Geometry: final body of the model. Coordinates: model frame, mm. A direction names the side the tool comes from. Give positions to 0.01 mm unless a question says otherwise; leave off trailing zeros. Order: outer loops, then holes, each group sorted by start corner. A loop starts at its lowest first (then second) coordinate and runs counter-clockwise, first axis right, second up. Notation, with made-up numbers: (-8, -5) -> (25, -5) arc R23 ccw to (25, 12) -> close; hole circle Ø4 at (48, -24). An arc over 180 degrees is marked (long way). Answer in a Markdown table with one row per item. Add a question column.
Q1. Cut plane C-C on z = 63. Return the cut outline in (x, y) (3 decimals), and give its area (3 significant figures).
Q2. Set-up query: faces 4 (the face through (25.4, 32, 6)), 5 (the face through (-12.827, 0, 63)), 6 (the face through (35, 25.4, 63)), 7 (the face through (-35, 25.4, 63)), 8 (the face through (38, 31, 118.745)). Return all of +Z, -Z, +X, -X, +Y, -Y with unobstructed straight access to the full face (end or side cutting, diameter ignored); none if empty.
Q3. Cut plane A-A on y = 2. Return the cut outline in (x, z).
Q4. Line query: line 1 along Z through (x, y) = (28.5, 60) (3 decimals); line 2 along X through (y, z) = (-3.5, 27); line 3 along X through (y, z) = (18, 77.5). Output: solid intervals per line, ascending. Write a range as from..to.
Q5. Pull-direction query (X, two-part tool) for faces 1 (the face through (0, 12.7, 63)), 2 (the face through (25.4, 32, 121)), 3 (the face through (-15, -12.7, 63)); classes: +X half, -X half, draft (parallel to the pull), parting line (faces both ways), or undercut.
Q6. Cut plane B-B on x = -38.5. Return the cut outline in (y, z) (3 decimals).
Q7. Contact query for flat-ended pins moving along their axis: P1, Ø1.5, axis at x = 40, z = 122.5, coming from the +Y side (3 decimals); P2, Ø5, axis at x = -31.5, z = 72, coming from the -Y side; P3, Ø7.5, axis at y = -1, z = 79, coming from the +X side. Output: stop coordinate, or through.
Q8. Cut plane D-D on x = 42. Return the cut outline in (y, z) (1 decimal), and give its area (3 significant figures).
from build123d import *

# Parameters (mm, degrees)
BOSS_EXTRUDE1_DEPTH = 127
SKETCH5_W           = 101.6
SKETCH5_H           = 127
BOSS_EXTRUDE3_DEPTH = 3.175
FILLET1_R           = 2.54
SKETCH6_W           = 101.6
SKETCH6_H           = 3.175
BOSS_EXTRUDE4_DEPTH = 101.6
BOSS_EXTRUDE6_DEPTH = 25.4
BOSS_EXTRUDE7_DEPTH = 0.254
BOSS_EXTRUDE8_DEPTH = 25.4
BOSS_EXTRUDE9_DEPTH = 0.254


with BuildPart() as part:
    # Sketch2 → Boss-Extrude1 (new body)
    with BuildSketch(Plane.XY):
        Polygon((-12.827, -12.7), (-16.637, -12.7), (-16.637, 25.4), (16.637, 25.4), (16.637, -12.7), (12.827, -12.7), (12.827, 12.7), (-12.827, 12.7), align=None)
    extrude(amount=BOSS_EXTRUDE1_DEPTH)

    # Sketch5 → Boss-Extrude3 (add)
    with BuildSketch(Plane(origin=(0, 25.4, 0), x_dir=(1, 0, 0), z_dir=(0, 1, 0))):
        with Locations((0, -63.5)):
            Rectangle(SKETCH5_W, SKETCH5_H)
    extrude(amount=BOSS_EXTRUDE3_DEPTH)

    # Fillet1
    fillet1_edges = [part.edges().sort_by_distance(p)[0] for p in [
        (-16.637, 25.4, 63.5),
        (16.637, 25.4, 63.5),
    ]]
    fillet(fillet1_edges, radius=FILLET1_R)

    # Sketch6 → Boss-Extrude4 (add)
    with BuildSketch(Plane(origin=(0, 28.575, 0), x_dir=(1, 0, 0), z_dir=(0, 1, 0))):
        with Locations((0, -125.4125)):
            Rectangle(SKETCH6_W, SKETCH6_H)
        with Locations((0, -1.5875)):
            Rectangle(SKETCH6_W, SKETCH6_H)
    extrude(amount=BOSS_EXTRUDE4_DEPTH)

    # Sketch9 → Boss-Extrude6 (add)
    with BuildSketch(Plane(origin=(50.8, 0, 0), x_dir=(0, 0, -1), z_dir=(1, 0, 0))):
        with BuildLine():
            Line((-123.825, 33.655), (-123.825, 29.9085))
            ThreePointArc((-123.825, 29.9085), (-121.548573107, 30.851426893), (-122.4915, 28.575))
            Line((-122.4915, 28.575), (-118.745, 28.575))
            Line((-118.745, 28.575), (-118.745, 33.655))
            Line((-118.745, 33.655), (-123.825, 33.655))
        make_face()
    extrude(amount=-BOSS_EXTRUDE6_DEPTH)

    # Sketch10 → Boss-Extrude7 (add)
    with BuildSketch(Plane(origin=(50.8, 0, 0), x_dir=(0, 0, -1), z_dir=(1, 0, 0))):
        with BuildLine():
            Line((-123.825, 29.9085), (-123.825, 28.575))
            Line((-123.825, 28.575), (-122.4915, 28.575))
            ThreePointArc((-122.4915, 28.575), (-121.548573107, 30.851426893), (-123.825, 29.9085))
        make_face()
    extrude(amount=-BOSS_EXTRUDE7_DEPTH)

    # Sketch17 → Boss-Extrude8 (add)
    with BuildSketch(Plane(origin=(50.8, 0, 0), x_dir=(0, 0, -1), z_dir=(1, 0, 0))):
        with BuildLine():
            Line((-8.255, 28.575), (-4.5085, 28.575))
            ThreePointArc((-4.5085, 28.575), (-5.451426893, 30.851426893), (-3.175, 29.9085))
            Line((-3.175, 29.9085), (-3.175, 33.655))
            Line((-3.175, 33.655), (-8.255, 33.655))
            Line((-8.255, 33.655), (-8.255, 28.575))
        make_face()
    extrude(amount=-BOSS_EXTRUDE8_DEPTH)

    # Sketch18 → Boss-Extrude9 (add)
    with BuildSketch(Plane(origin=(50.8, 0, 0), x_dir=(0, 0, -1), z_dir=(1, 0, 0))):
        with BuildLine():
            Line((-3.175, 29.9085), (-3.175, 28.575))
            Line((-3.175, 28.575), (-4.5085, 28.575))
            ThreePointArc((-4.5085, 28.575), (-5.451426893, 30.851426893), (-3.175, 29.9085))
        make_face()
    extrude(amount=-BOSS_EXTRUDE9_DEPTH)


solid = part.part
Completed:
| question | item | result |
|---|---|---|
| 1 | outline | (-50.8, 25.4) -> (-19.177, 25.4) arc R2.54 cw to (-16.637, 22.86) -> (-16.637, -12.7) -> (-12.827, -12.7) -> (-12.827, 12.7) -> (12.827, 12.7) -> (12.827, -12.7) -> (16.637, -12.7) -> (16.637, 22.86) arc R2.54 cw to (19.177, 25.4) -> (50.8, 25.4) -> (50.8, 28.575) -> (-50.8, 28.575) -> close |
| 1 | area | 941 mm² |
| 2 | face 4 | -X, +Y |
| 2 | face 5 | +Z, -Z, -Y |
| 2 | face 6 | +Z, -Z, +X, -Y |
| 2 | face 7 | +Z, -Z, -X, -Y |
| 2 | face 8 | +X, -X, +Y |
| 3 | outline | (-16.64, 0) -> (-12.83, 0) -> (-12.83, 127) -> (-16.64, 127) -> close; (12.83, 0) -> (16.64, 0) -> (16.64, 127) -> (12.83, 127) -> close |
| 4 | line 1 | z = 0..3.175, 123.825..127 |
| 4 | line 2 | x = -16.64..-12.83, 12.83..16.64 |
| 4 | line 3 | x = -16.64..16.64 |
| 5 | face 1 | undercut |
| 5 | face 2 | -X half |
| 5 | face 3 | draft |
| 6 | outline | (25.4, 0) -> (130.175, 0) -> (130.175, 3.175) -> (28.575, 3.175) -> (28.575, 123.825) -> (130.175, 123.825) -> (130.175, 127) -> (25.4, 127) -> close |
| 7 | P1 | stops at y = 33.655 |
| 7 | P2 | stops at y = 25.4 |
| 7 | P3 | stops at x = 16.64 |
| 8 | outline | (25.4, 0) -> (130.2, 0) -> (130.2, 3.2) -> (33.7, 3.2) -> (33.7, 8.3) -> (28.6, 8.3) -> (28.6, 118.7) -> (33.7, 118.7) -> (33.7, 123.8) -> (130.2, 123.8) -> (130.2, 127) -> (25.4, 127) -> close; hole (28.6, 3.2) -> (29.9, 3.2) arc R1.3 ccw (long way) to (28.6, 4.5) -> close; hole (28.6, 122.5) arc R1.3 ccw (long way) to (29.9, 123.8) -> (28.6, 123.8) -> close |
| 8 | area | 1,090 mm² |
